Verification items for the finished model (mm, model axes). Face numbers are marked on the shaded views. A direction names the side the tool comes from. Round coordinates to 2 decimals unless told otherwise and drop trailing zeros. Write each loop counter-clockwise with the first axis right and the second up, starting at its lowest first coordinate (ties: lowest second). Pieces come first, ordered by that corner, then holes.
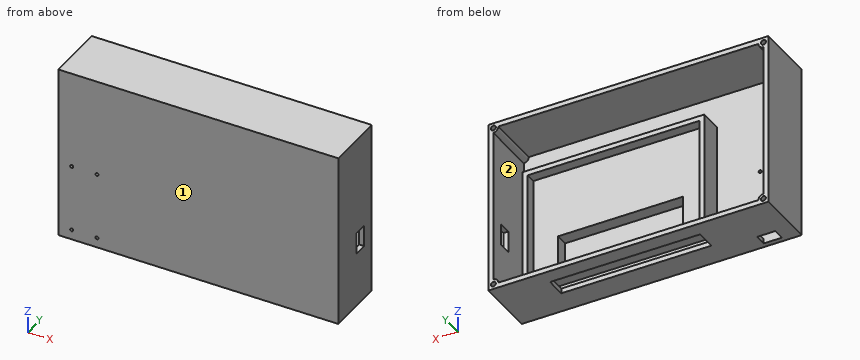
from build123d import *

# Parameters (mm, degrees)
SKETCH1_W           = 168
SKETCH1_H           = 105
BOSS_EXTRUDE1_DEPTH = 35.5
SHELL3_T            = -3
SKETCH3_R           = 0.925
CUT_EXTRUDE2_DEPTH  = 3
SKETCH7_W           = 109
SKETCH7_H           = 69
SKETCH7_W_2         = 103
SKETCH7_H_2         = 63
BOSS_EXTRUDE3_DEPTH = 13.6
SKETCH8_W           = 103
SKETCH8_H           = 63
SKETCH8_W_2         = 75
SKETCH8_H_2         = 20
BOSS_EXTRUDE4_DEPTH = 7.5
SKETCH2_W           = 11
SKETCH2_H           = 7
SKETCH2_W_2         = 90
SKETCH2_H_2         = 12
CUT_EXTRUDE1_DEPTH  = 3
BOSS_EXTRUDE2_DEPTH = 32.5
SKETCH5_R           = 1.5
CUT_EXTRUDE3_DEPTH  = 29.5
SKETCH13_W          = 13
SKETCH13_H          = 8
CUT_EXTRUDE8_DEPTH  = 3


with BuildPart() as part:
    # Sketch1 → Boss-Extrude1 (new body)
    with BuildSketch(Plane(origin=(0, 0, 0), x_dir=(1, 0, 0), z_dir=(0, 1, 0))):
        with Locations((84, 52.5)):
            Rectangle(SKETCH1_W, SKETCH1_H)
    extrude(amount=BOSS_EXTRUDE1_DEPTH)

    # Shell3
    shell3_openings = [part.faces().sort_by_distance(p)[0] for p in [
        (84, 35.5, -52.5),
    ]]
    offset(amount=SHELL3_T, openings=shell3_openings, kind=Kind.INTERSECTION)

    # Sketch3 → Cut-Extrude2 (cut)
    with BuildSketch(Plane(origin=(0, 3, 0), x_dir=(1, 0, 0), z_dir=(0, 1, 0))):
        with Locations((8, 99)):
            Circle(SKETCH3_R)
        with Locations((23.23, 99)):
            Circle(SKETCH3_R)
        with Locations((23.23, 58.76)):
            Circle(SKETCH3_R)
        with Locations((8, 58.76)):
            Circle(SKETCH3_R)
    extrude(amount=-CUT_EXTRUDE2_DEPTH, mode=Mode.SUBTRACT)

    # Sketch7 → Boss-Extrude3 (add)
    with BuildSketch(Plane(origin=(0, 3, 0), x_dir=(1, 0, 0), z_dir=(0, 1, 0))):
        with Locations((103.5, 56.5)):
            Rectangle(SKETCH7_W, SKETCH7_H)
        with Locations((103.5, 56.5)):
            Rectangle(SKETCH7_W_2, SKETCH7_H_2, mode=Mode.SUBTRACT)
    extrude(amount=BOSS_EXTRUDE3_DEPTH)

    # Sketch8 → Boss-Extrude4 (add)
    with BuildSketch(Plane(origin=(0, 3, 0), x_dir=(1, 0, 0), z_dir=(0, 1, 0))):
        with Locations((103.5, 56.5)):
            Rectangle(SKETCH8_W, SKETCH8_H)
        with Locations((102.8, 75)):
            Rectangle(SKETCH8_W_2, SKETCH8_H_2, mode=Mode.SUBTRACT)
    extrude(amount=BOSS_EXTRUDE4_DEPTH)

    # Sketch2 → Cut-Extrude1 (cut)
    with BuildSketch(Plane(origin=(0, 0, -105), x_dir=(-1, 0, 0), z_dir=(0, 0, -1))):
        with Locations((-15.615, 6.5)):
            Rectangle(SKETCH2_W, SKETCH2_H)
        with Locations((-91, 20.6)):
            Rectangle(SKETCH2_W_2, SKETCH2_H_2)
    extrude(amount=-CUT_EXTRUDE1_DEPTH, mode=Mode.SUBTRACT)

    # Sketch4 → Boss-Extrude2 (add)
    with BuildSketch(Plane(origin=(0, 3, 0), x_dir=(1, 0, 0), z_dir=(0, 1, 0))):
        with BuildLine():
            Line((6, 102), (3, 102))
            Line((3, 102), (3, 99))
            ThreePointArc((3, 99), (5.121320344, 99.878679656), (6, 102))
        make_face()
        with BuildLine():
            Line((162, 102), (165, 102))
            Line((165, 102), (165, 99))
            ThreePointArc((165, 99), (162.878679656, 99.878679656), (162, 102))
        make_face()
        with BuildLine():
            Line((165, 3), (165, 6))
            ThreePointArc((165, 6), (162.878679656, 5.121320344), (162, 3))
            Line((162, 3), (165, 3))
        make_face()
        with BuildLine():
            Line((6, 3), (3, 3))
            Line((3, 3), (3, 6))
            ThreePointArc((3, 6), (5.121320344, 5.121320344), (6, 3))
        make_face()
    extrude(amount=BOSS_EXTRUDE2_DEPTH)

    # Sketch5 → Cut-Extrude3 (cut)
    with BuildSketch(Plane(origin=(0, 35.5, 0), x_dir=(1, 0, 0), z_dir=(0, 1, 0))):
        with Locations((3, 102)):
            Circle(SKETCH5_R)
        with Locations((165, 102)):
            Circle(SKETCH5_R)
        with Locations((3, 3)):
            Circle(SKETCH5_R)
        with Locations((165, 3)):
            Circle(SKETCH5_R)
    extrude(amount=-CUT_EXTRUDE3_DEPTH, mode=Mode.SUBTRACT)

    # Sketch13 → Cut-Extrude8 (cut)
    with BuildSketch(Plane(origin=(168, 0, 0), x_dir=(0, 0, -1), z_dir=(1, 0, 0))):
        with Locations((65.5, 23.5)):
            Rectangle(SKETCH13_W, SKETCH13_H)
    extrude(amount=-CUT_EXTRUDE8_DEPTH, mode=Mode.SUBTRACT)


solid = part.part
Q1. Depth check by flat-ended pin: P1, Ø1, axis at x = 99, y = 20.5, coming from the -Z side; P2, Ø0.9, axis at x = 165.5, z = -102, coming from the +Y side; P3, Ø2, axis at x = 80.5, z = -24.5, coming from the +Y side. Enter the tip coordinate at first touch or a pass-through.
Recorded:
P1: stops at z = -3
P2: stops at y = 6
P3: stops at y = 16.6
Q2. Tool access check on the marked faces 1 and 2. Record the directions out of +Z, -Z, +X, -X, +Y, -Y that give a thin tool (end or side, any length) a straight path to the whole face; none if there is none.
Recorded:
face 1: +Z, -Z, +X, -X, -Y
face 2: +Y
Q3. Sectioned sample at A-A (y = 24.5). Enter the section's corners in (x, z).
Recorded:
outline: (0, -105) - (46, -105) - (46, -102) - (6, -102) arc R3 ccw to (3, -99) - (3, -6) arc R3 ccw to (6, -3) - (162, -3) arc R3 ccw to (165, -6) - (165, -59) - (168, -59) - (168, 0) - (0, 0) - close; (136, -105) - (168, -105) - (168, -72) - (165, -72) - (165, -99) arc R3 ccw to (162, -102) - (136, -102) - close; hole circle Ø3 at (3, -102); hole circle Ø3 at (3, -3); hole circle Ø3 at (165, -102); hole circle Ø3 at (165, -3)
Q4. Sectioned sample at B-B (x = 89). Enter the section's corners in (y, z).
Recorded:
outline: (0, -105) - (14.6, -105) - (14.6, -102) - (3, -102) - (3, -91) - (16.6, -91) - (16.6, -88) - (10.5, -88) - (10.5, -85) - (3, -85) - (3, -65) - (10.5, -65) - (10.5, -25) - (16.6, -25) - (16.6, -22) - (3, -22) - (3, -3) - (35.5, -3) - (35.5, 0) - (0, 0) - close; (26.6, -105) - (35.5, -105) - (35.5, -102) - (26.6, -102) - close
Q5. Sectioned sample at C-C (z = -82). Enter the section's corners in (x, y), plus the area to 3 significant figures.
Recorded:
outline: (0, 0) - (168, 0) - (168, 35.5) - (165, 35.5) - (165, 3) - (158, 3) - (158, 16.6) - (155, 16.6) - (155, 10.5) - (140.3, 10.5) - (140.3, 3) - (65.3, 3) - (65.3, 10.5) - (52, 10.5) - (52, 16.6) - (49, 16.6) - (49, 3) - (3, 3) - (3, 35.5) - (0, 35.5) - close
area: 991 mm2
Q6. Material ranges on line 1 along Z through (x, y) = (58, 12.5); line 2 along Z through (x, y) = (8, 1.45) (3 decimals); line 3 along X through (y, z) = (1, -99) (3 decimals), recorded low to high.
Recorded:
line 1: z = -105 to -102, -91 to -88, -25 to -22, -3 to 0
line 2: z = -105 to -99.925, -98.075 to -59.685, -57.835 to 0
line 3: x = 0 to 7.075, 8.925 to 22.305, 24.155 to 168
Q7. Sectioned sample at D-D (x = 144). Enter the section's corners in (y, z).
Recorded:
outline: (0, -105) - (35.5, -105) - (35.5, -102) - (3, -102) - (3, -91) - (16.6, -91) - (16.6, -88) - (10.5, -88) - (10.5, -25) - (16.6, -25) - (16.6, -22) - (3, -22) - (3, -3) - (35.5, -3) - (35.5, 0) - (0, 0) - close
